```python
from build123d import *

# Parameters (mm, degrees)
CROQUIS1_W                   = 20
CROQUIS1_H                   = 20
SALIENTE_EXTRUIR1_DEPTH      = 3
TALADRO_DE_MARGEN_PARA_M52_D = 5.5
CORTAR_EXTRUIR1_DEPTH        = 3


with BuildPart() as part:
    # Croquis1 → Saliente-Extruir1 (new body)
    with BuildSketch(Plane.XY):
        with BuildLine():
            Line((-143.5, 0), (143.5, 0))
            Line((143.5, 0), (143.5, 30))
            Line((143.5, 30), (9.355173022, 385.226719524))
            ThreePointArc((9.355173022, 385.226719524), (0, 391.693910765), (-9.355173022, 385.226719524))
            Line((-9.355173022, 385.226719524), (-143.5, 30))
            Line((-143.5, 30), (-143.5, 0))
        make_face()
        with Locations((0, 365)):
            Rectangle(CROQUIS1_W, CROQUIS1_H, mode=Mode.SUBTRACT)
        with Locations((0, 335)):
            Rectangle(CROQUIS1_W, CROQUIS1_H, mode=Mode.SUBTRACT)
    extrude(amount=SALIENTE_EXTRUIR1_DEPTH)

    # Taladro de margen para M52 (through all)
    with Locations(Plane(origin=(0, 0, 0), x_dir=(-1, 0, 0), z_dir=(0, 0, -1))):
        with Locations((-85, 15), (85, 15)):
            Hole(TALADRO_DE_MARGEN_PARA_M52_D / 2)

    # Croquis4 → Cortar-Extruir1 (cut)
    with BuildSketch(Plane(origin=(0, 0, 0), x_dir=(-1, 0, 0), z_dir=(0, 0, -1))):
        with BuildLine():
            Line((9.355173022, 250.226719524), (74.889584061, 76.686118864))
            ThreePointArc((74.889584061, 76.686118864), (73.760226731, 67.466838773), (65.534411039, 63.153310105))
            Line((65.534411039, 63.153310105), (-65.534411039, 63.153310105))
            ThreePointArc((-65.534411039, 63.153310105), (-73.760226731, 67.466838773), (-74.889584061, 76.686118864))
            Line((-74.889584061, 76.686118864), (-9.355173022, 250.226719524))
            ThreePointArc((-9.355173022, 250.226719524), (0, 256.693910765), (9.355173022, 250.226719524))
        make_face()
    extrude(amount=-CORTAR_EXTRUIR1_DEPTH, mode=Mode.SUBTRACT)


solid = part.part
```
Geometry: final body of the model. Coordinates: model frame, mm. A direction names the side the tool comes from. Coordinates: 2 decimals unless noted, no trailing zeros. Order: outer loops, then holes, each group sorted by start corner. A loop starts at its lowest first (then second) coordinate and runs counter-clockwise, first axis right, second up. Notation, with made-up numbers: (37.25, 52.25) - (85.25, 52.25) arc R16 cw to (85.25, 69.25) - close; hole circle Ø4 at (26, -14.5). An arc over 180 degrees is marked (long way). Write each question's results on one line, items separated by ' | '.
1) Pin query (flat end, axial travel): pin 1 (0.9 mm diameter, centred on x = -4.5, z = 2, fed in from +Y); pin 2 (1.5 mm diameter, centred on x = 7, z = 2, fed in from +Y); pin 3 (0.9 mm diameter, centred on x = 4, z = 1, fed in from +Y). Return the tip coordinate at first contact, or that it passes through.
Results list:
pin 1: y = 390.84 | pin 2: y = 389.5 | pin 3: y = 391.04
2) Section B-B, the plane y = 144. Return loops of the section in (x, z), plus the area to 3 significant figures.
Results list:
outline: (-100.45, 0) - (-49.47, 0) - (-49.47, 3) - (-100.45, 3) - close; (49.47, 0) - (100.45, 0) - (100.45, 3) - (49.47, 3) - close | area: 306 mm^2
3) Section C-C, the plane z = 2.1. Return loops of the section in (x, y).
Results list:
outline: (-143.5, 0) - (143.5, 0) - (143.5, 30) - (9.36, 385.23) arc R10 ccw to (-9.36, 385.23) - (-143.5, 30) - close; hole circle Ø5.5 at (-85, 15); hole (-74.89, 76.69) arc R10 ccw to (-65.53, 63.15) - (65.53, 63.15) arc R10 ccw to (74.89, 76.69) - (9.36, 250.23) arc R10 ccw to (-9.36, 250.23) - close; hole (-10, 325) - (10, 325) - (10, 345) - (-10, 345) - close; hole (-10, 355) - (10, 355) - (10, 375) - (-10, 375) - close; hole circle Ø5.5 at (85, 15)
4) Set-up query: faces 1 (the flat face through (42.58, 162.24, 1.48)), 2 (the flat face through (62, 155, 3)). Return all of +Z, -Z, +X, -X, +Y, -Y with unobstructed straight access to the full face (end or side cutting, diameter ignored); none if empty.
Results list:
face 1: +Z, -Z | face 2: +Z, +X, -X, +Y, -Y
5) Section D-D, the plane y = 301. Return loops of the section in (x, z).
Results list:
outline: (-41.16, 0) - (41.16, 0) - (41.16, 3) - (-41.16, 3) - close
6) Pull-direction query (Y, two-part tool) for faces 3 (the flat face through (62, 155, 0)), 4 (the flat face through (77.367, 205.127, 1.479)), 5 (the flat face through (-41.664, 164.671, 1.479)); classes: pulls with the +Y half, pulls with the -Y half, needs draft (parallel to the pull), parting line crosses it, or undercut.
Results list:
face 3: needs draft | face 4: pulls with the +Y half | face 5: undercut
7) Section A-A, the plane x = 48. Return loops of the section in (y, z), plus the area to 3 significant figures.
Results list:
outline: (0, 0) - (63.15, 0) - (63.15, 3) - (0, 3) - close; (147.89, 0) - (282.89, 0) - (282.89, 3) - (147.89, 3) - close | area: 594 mm^2
8) Line query: line 1 (Y direction, x = -6, z = 2.6); line 2 (X direction, y = 357.5, z = 1.45); line 3 (X direction, y = 194, z = 0.1). Output: solid intervals per line, ascending. Write a range as from..to.
Results list:
line 1: 0..63.15, 254.69..325, 345..355, 375..389.69 | line 2: -19.83..-10, 10..19.83 | line 3: -81.57..-30.59, 30.59..81.57
